Autodesk Inventor part; units mm, degrees
ref_plane "YZ Plane" through (0, 0, 0) normal (1, 0, 0) x (0, 1, 0)
ref_plane "XZ Plane" through (0, 0, 0) normal (0, 1, 0) x (-1, 0, 0)
ref_plane "XY Plane" through (0, 0, 0) normal (0, 0, 1) x (1, 0, 0)
sketch "Skizze5" plane through (0, 0, 0) normal (0, 1, 0) x (-1, 0, 0)
  line L0 (0, 0) -> (-310, 0)
  line L1 (-310, 0) -> (-310, -310)
  line L2 (-310, -310) -> (0, -310)
  line L3 (0, -310) -> (0, 0)
  dimension "d14" = 310
  dimension "d15" = 310
extrude "Extrusion5" add sketch "Skizze5" along normal blind 500
sketch "Skizze6" plane through (0, 500, 0) normal (0, 1, 0) x (1, 0, 0)
  line L0 (0, 310) -> (0, 0)
  line L1 (0, 0) -> (310, 0)
  line L2 (40, 35) -> (270, 35)
  line L3 (270, 35) -> (270, 0)
  line L4 (270, 0) -> (40, 0)
  line L5 (40, 0) -> (40, 35)
  dimension "d20" = 230
extrude "Extrusion6" cut sketch "Skizze6" against normal blind 500
sketch "Skizze7" plane through (0, 0, 0) normal (0, -1, 0) x (1, 0, 0)
  line L0 (310, 0) -> (310, -310)
  line L1 (40, -35) -> (270, -35)
  line L2 (310, 0) -> (270, 0)
  line L3 (270, 0) -> (270, -35)
  line L4 (270, -35) -> (310, -35)
  line L5 (310, -35) -> (310, 0)
  line L6 (40, 0) -> (40, -35)
  line L7 (0, -310) -> (0, 0)
  line L8 (40, 0) -> (0, 0)
  line L9 (0, 0) -> (0, -35)
  line L10 (0, -35) -> (40, -35)
  line L11 (40, -35) -> (40, 0)
  line L12 (310, -35) -> (0, -35)
  line L13 (0, -35) -> (0, -285)
  line L14 (0, -285) -> (310, -285)
  line L15 (310, -285) -> (310, -35)
  line L16 (310, -310) -> (0, -310)
  line L17 (310, -285) -> (285, -285)
  line L18 (285, -285) -> (285, -310)
  line L19 (285, -310) -> (310, -310)
  line L20 (310, -310) -> (310, -285)
  line L21 (0, -285) -> (25, -285)
  line L22 (25, -285) -> (25, -310)
  line L23 (25, -310) -> (0, -310)
  line L24 (0, -310) -> (0, -285)
  dimension "d23" = 250
  dimension "d24" = 25
  dimension "d25" = 25
extrude "Extrusion7" cut sketch "Skizze7" against normal blind 480 contours L0 L4 L3 L2 | L0 L14 L7 L10 L1 L4 | L18 L16 L22 L14 | L10 L7 L8 L6
sketch "Skizze8" plane through (0, 500, 0) normal (0, 1, 0) x (1, 0, 0)
  line L0 (0, 0) -> (40, 0)
  circle A0 centre (155, 155) radius 36
  dimension "d30" = 72
extrude "Extrusion8" cut sketch "Skizze8" against normal blind 20
sketch "Skizze9" plane through (0, 480, 0) normal (0, -1, 0) x (1, 0, 0)
  point P0 (0, 0)
sketch "Skizze10" plane through (0, 480, 0) normal (0, -1, 0) x (1, 0, 0)
  line L0 (270, 0) -> (310, 0)
  line L1 (270, 0) -> (275, 0)
  line L2 (275, 0) -> (275, -35)
  line L3 (275, -35) -> (270, -35)
  line L4 (270, -35) -> (270, 0)
  line L5 (39.9329, 0) -> (34.9329, 0)
  line L6 (34.9329, 0) -> (34.9329, -35)
  line L7 (34.9329, -35) -> (39.9329, -35)
  line L8 (39.9329, -35) -> (39.9329, 0)
  point P0 (0, 0)
  dimension "d33" = 5
  dimension "d34" = 35
  dimension "d35" = 5
extrude "Extrusion9" add sketch "Skizze10" along normal blind 30
sketch "Skizze11" plane through (0, 500, 0) normal (0, 0, 1) x (1, 0, 0)
  line L0 (0, -20) -> (0, 0)
  line L1 (0, -20) -> (34.9329, -20)
  line L2 (0, -20) -> (34.9329, -20)
  line L3 (39.9329, -50) -> (34.9329, -50)
  line L4 (34.9329, -20) -> (34.9329, -50)
  line L5 (34.9329, -50) -> (0, -20)
  line L6 (275, -20) -> (310, -20)
  line L7 (310, -20) -> (275, -20)
  line L8 (275, -20) -> (275, -50)
  line L9 (275, -20) -> (275, -50)
  line L10 (275, -50) -> (310, -20)
  point P0 (0, -500)
extrude "Extrusion10" add sketch "Skizze11" against normal blind 5
sketch "Skizze12" plane through (34.9329, 450, -35) normal (-1, 0, 0) x (0, 0, 1)
  line L0 (30, 0) -> (0, 0)
  line L1 (0, 0) -> (15, 0)
  line L2 (15, 0) -> (15, 15)
  line L3 (15, 15) -> (0, 15)
  line L4 (0, 15) -> (0, 0)
  point P0 (35, -450)
  dimension "d40" = 15
  dimension "d41" = 15
hole "Bohrung1" at (34.9329, 465, -20) direction (1, 0, 0) diameter 10 depth 27.3 tip angle 118
sketch "Skizze13" plane through (275, 450, -35) normal (1, 0, 0) x (0, 0, -1)
  line L0 (0, 0) -> (-15, 0)
  line L1 (-15, 0) -> (-15, 15)
  line L2 (-15, 15) -> (0, 15)
  line L3 (0, 15) -> (0, 0)
  point P0 (-35, -450)
  dimension "d49" = 15
  dimension "d50" = 15
hole "Bohrung2" at (275, 465, -20) direction (-1, 0, 0) diameter 10 depth 27.3 tip angle 118
chamfer "Fase1" distance 2 angle 45 1 edges at (34.9329, 465, -25)
chamfer "Fase2" distance 2 angle 45 1 edges at (275, 465, -15)
sketch "Skizze14" plane through (0, 500, 0) normal (0, 1, 0) x (1, 0, 0)
  line L0 (310, 0) -> (310, 310)
  line L1 (310, 310) -> (297.5, 310)
  line L2 (297.5, 310) -> (297.5, 297.5)
  line L3 (297.5, 297.5) -> (310, 297.5)
  line L4 (310, 297.5) -> (310, 310)
  line L5 (0, 310) -> (0, 285)
  line L6 (0, 310) -> (12.5, 310)
  line L7 (12.5, 310) -> (12.5, 297.5)
  line L8 (12.5, 297.5) -> (0, 297.5)
  line L9 (0, 297.5) -> (0, 310)
  point P0 (0, 0)
  dimension "d64" = 12.5
  dimension "d65" = 12.5
  dimension "d66" = 12.5
  dimension "d67" = 12.5
hole "Bohrung3" at (12.5, 500, -297.5) at (297.5, 500, -297.5) direction (0, -1, 0) diameter 10 depth 27.3 tip angle 118
chamfer "Fase3" distance 2 angle 45 2 edges at (297.5, 500, -302.5) (12.5, 500, -302.5)
properties part number "Haltung_Presse"
Here's how the part is built. I have some questions about the finished solid (model axes, mm). A direction names the side the tool comes from. Round coordinates to 2 decimals unless told otherwise and drop trailing zeros. Order: outer loops, then holes, each group sorted by start corner. A loop starts at its lowest first (then second) coordinate and runs counter-clockwise, first axis right, second up. Notation, with made-up numbers: M 35,38 L 49,38 A20 cw 49,72 Z; hole C 47,21.5 d4. An arc over 180 degrees is marked long. One line per question, with ' | ' between items.
1) For faces 5 (the face through (153, 490, -35)), 6 (the face through (292.255, 464.79, -2.465)), 7 (the face through (293.284, 485.173, -294.812)), which set-ups out of +Z, -Z, +X, -X, +Y, -Y let a thin tool reach every point of the face, with its end or its side?
Working result:
face 5: +Z, +Y, -Y | face 6: +Z, +X, -Y | face 7: +Y
2) I want a section at B-B, the plane y = 102.5. Write out the boundary of the cut face in (x, z).
Working result:
outline: M 0,-310 L 25,-310 L 25,-285 L 0,-285 Z; M 285,-310 L 310,-310 L 310,-285 L 285,-285 Z
3) I want a section at D-D, the plane z = -225. Write out the boundary of the cut face in (x, y).
Working result:
outline: M 0,480 L 310,480 L 310,500 L 0,500 Z
4) If we mould it in two halves opening along X, with no side actions, what happens to faces 1 (the face through (273.125, 470.081, -19.333)), 2 (the face through (12.54, 470.22, -298.37)), 3 (the face through (299.039, 498.125, -292.612)), 4 (the face through (25, 472, -5))? For each: +X half, -X half, draft (parallel to the pull), parting line (faces both ways), or undercut.
Working result:
face 1: +X half | face 2: undercut | face 3: undercut | face 4: draft
5) For pin 1 Ø9 at (x, z) = (297.5, -297.5) entering from +Y; pin 2 Ø4 at (x, z) = (271.5, -16.5) entering from -Y; pin 3 Ø15 at (y, z) = (469, -19) entering from +X, each with a flat end and sliding along its axis, tell me the tip position at first contact or that it passes through.
Working result:
pin 1: y = 472.4 | pin 2: y = 450 | pin 3: x = 275
6) I want a section at C-C, the plane x = 212. Write out the boundary of the cut face in (y, z), then the cut area to 3 significant figures.
Working result:
outline: M 480,-310 L 500,-310 L 500,-35 L 480,-35 Z | area: 5,500 mm²
7) I want a section at A-A, the plane z = -155. Write out the boundary of the cut face in (x, y), then the cut area to 3 significant figures.
Working result:
outline: M 0,480 L 119,480 L 119,500 L 0,500 Z; M 191,480 L 310,480 L 310,500 L 191,500 Z | area: 4,760 mm²
8) I need wall thicknesses on line 1 along Y through (x, z) = (37.7, -20); line 2 along X through (y, z) = (200.5, -290.5); line 3 along Z through (x, y) = (12, 484). Which ranges of each line are inside material? Lowest first, please.
Working result:
line 1: 450 to 460, 470 to 500 | line 2: 0 to 25, 285 to 310 | line 3: -310 to -302.47, -292.53 to 0
